Can you work these out from the model? Positions are in its coordinate system, mm. A direction names the side the tool comes from. Coordinates: 2 decimals unless noted, no trailing zeros. Order: outer loops, then holes, each group sorted by start corner. A loop starts at its lowest first (then second) coordinate and runs counter-clockwise, first axis right, second up.
```python
from build123d import *

# Parameters (mm, degrees)
SKETCH1_R                = 72.8
SKETCH1_R_2              = 2.065
SKETCH1_R_3              = 1.9558
SKETCH1_R_4              = 33.25
BOSS_EXTRUDE1_DEPTH      = 3.175
BOSS_EXTRUDE4_START      = 20
SKETCH14_R               = 72.8
SKETCH14_R_2             = 52.8
BOSS_EXTRUDE4_DEPTH      = 20
SKETCH15_R               = 2.065
CUT_EXTRUDE6_DEPTH       = 106.530851532
M5_CLEARANCE_HOLE1_D     = 5.3
CUT_EXTRUDE8_DEPTH       = 106.530851532
FILLET1_R                = 5
CIRPATTERN4_COUNT        = 3
FILLET1_OF_CIRPATTERN4_R = 5
BOSS_EXTRUDE8_START      = -20.175
BOSS_EXTRUDE8_DEPTH      = 30.175
CUT_EXTRUDE9_START       = -10
CUT_EXTRUDE9_DEPTH       = 10
CIRPATTERN5_COUNT        = 3


with BuildPart() as part:
    # Sketch1 → Boss-Extrude1 (new body)
    with BuildSketch(Plane.XY):
        Circle(SKETCH1_R)
        with Locations((50.662486121, -29.25)):
            Circle(SKETCH1_R_2, mode=Mode.SUBTRACT)
        with Locations((59.322740159, -34.25)):
            Circle(SKETCH1_R_2, mode=Mode.SUBTRACT)
        with Locations((-59.322740159, -34.25)):
            Circle(SKETCH1_R_2, mode=Mode.SUBTRACT)
        with Locations((-50.662486121, -29.25)):
            Circle(SKETCH1_R_2, mode=Mode.SUBTRACT)
        with Locations((0, 44.45)):
            Circle(SKETCH1_R_3, mode=Mode.SUBTRACT)
        with Locations((-44.45, 0)):
            Circle(SKETCH1_R_3, mode=Mode.SUBTRACT)
        with Locations((0, -44.45)):
            Circle(SKETCH1_R_3, mode=Mode.SUBTRACT)
        with Locations((31.430896424, -31.430896424)):
            Circle(SKETCH1_R_3, mode=Mode.SUBTRACT)
        with Locations((44.45, 0)):
            Circle(SKETCH1_R_3, mode=Mode.SUBTRACT)
        with Locations((0, 68.5)):
            Circle(SKETCH1_R_2, mode=Mode.SUBTRACT)
        with Locations((0, 58.5)):
            Circle(SKETCH1_R_2, mode=Mode.SUBTRACT)
        Circle(SKETCH1_R_4, mode=Mode.SUBTRACT)
    extrude(amount=BOSS_EXTRUDE1_DEPTH)

    # Sketch14 → Boss-Extrude4 (add)
    with BuildSketch(Plane(origin=(0, 0, 0), x_dir=(-1, 0, 0), z_dir=(0, 0, -1)).offset(BOSS_EXTRUDE4_START)):
        Circle(SKETCH14_R)
        Circle(SKETCH14_R_2, mode=Mode.SUBTRACT)
    extrude(amount=-BOSS_EXTRUDE4_DEPTH)

    # Sketch15 → Cut-Extrude6 (cut, through all)
    with BuildSketch(Plane.XY.offset(3.175)):
        with Locations((-59.322740159, -34.25)):
            Circle(SKETCH15_R)
        with Locations((-50.662486121, -29.25)):
            Circle(SKETCH15_R)
        with Locations((59.322740159, -34.25)):
            Circle(SKETCH15_R)
        with Locations((50.662486121, -29.25)):
            Circle(SKETCH15_R)
        with Locations((0, 58.5)):
            Circle(SKETCH15_R)
        with Locations((0, 68.5)):
            Circle(SKETCH15_R)
    extrude(amount=-CUT_EXTRUDE6_DEPTH, mode=Mode.SUBTRACT)

    # M5 Clearance Hole1 (through all)
    with Locations(Plane.XY.offset(3.175)):
        with Locations((0, 58.5), (0, 68.5), (50.662486121, -29.25), (59.322740159, -34.25), (-59.322740159, -34.25), (-50.662486121, -29.25)):
            Hole(M5_CLEARANCE_HOLE1_D / 2)

    # Sketch30 → Cut-Extrude8 (cut, through all)
    with BuildSketch(Plane(origin=(0, 0, -20), x_dir=(-1, 0, 0), z_dir=(0, 0, -1))):
        with BuildLine():
            ThreePointArc((-21.891382204, 69.430594014), (-63.046649396, 36.4), (-71.074349318, -15.756803895))
            Line((-71.074349318, -15.756803895), (-56.429909212, -12.510209686))
            Line((-56.429909212, -12.510209686), (-54.477317197, -12.077330458))
            ThreePointArc((-54.477317197, -12.077330458), (-48.324217531, 27.9), (-16.779383612, 53.217405852))
            Line((-16.779383612, 53.217405852), (-17.380795211, 55.124839753))
            Line((-17.380795211, 55.124839753), (-21.891382204, 69.430594014))
        make_face()
    cut_extrude8 = extrude(amount=-CUT_EXTRUDE8_DEPTH, mode=Mode.SUBTRACT)

    # Fillet1
    fillet1_edges = [part.edges().sort_by_distance(p)[0] for p in [
        (54.477317197, -12.077330458, -8.4125),
        (16.779383612, 53.217405852, -8.4125),
    ]]
    fillet(fillet1_edges, radius=FILLET1_R)

    # CirPattern4: Cut-Extrude8 ×3 about axis
    cirpattern4_axis = Axis((0, 0, 0), (0, 0, 1))
    for i in range(1, CIRPATTERN4_COUNT):
        add(cut_extrude8.rotate(cirpattern4_axis, i * 360 / CIRPATTERN4_COUNT), mode=Mode.SUBTRACT)

    # Fillet1 of CirPattern4
    fillet1_of_cirpattern4_edges = [part.edges().sort_by_distance(p)[0] for p in [
        (-16.779383612, 53.217405852, -8.4125),
        (-54.477317197, -12.077330458, -8.4125),
        (-37.697933585, -41.140075394, -8.4125),
        (37.697933585, -41.140075394, -8.4125),
    ]]
    fillet(fillet1_of_cirpattern4_edges, radius=FILLET1_OF_CIRPATTERN4_R)

    # Sketch31 → Boss-Extrude8 (add)
    with BuildSketch(Plane.XY.offset(3.175).offset(BOSS_EXTRUDE8_START)):
        with BuildLine():
            Line((21.891382204, 69.430594014), (21.816905179, 69.19438307))
            ThreePointArc((21.816905179, 69.19438307), (0, 72.552325945), (-21.816905179, 69.19438307))
            Line((-21.816905179, 69.19438307), (-22.883711342, 72.577859952))
            ThreePointArc((-22.883711342, 72.577859952), (0, 76.1), (22.883711342, 72.577859952))
            Line((22.883711342, 72.577859952), (21.891382204, 69.430594014))
        make_face()
    boss_extrude8 = extrude(amount=BOSS_EXTRUDE8_DEPTH)

    # Sketch32 → Cut-Extrude9 (cut)
    with BuildSketch(Plane.XY.offset(13.175).offset(CUT_EXTRUDE9_START)):
        with BuildLine():
            Line((21.816905179, 69.19438307), (22.883711342, 72.577859952))
            ThreePointArc((22.883711342, 72.577859952), (0, 76.1), (-22.883711342, 72.577859952))
            Line((-22.883711342, 72.577859952), (-21.816905179, 69.19438307))
            ThreePointArc((-21.816905179, 69.19438307), (0, 72.552325945), (21.816905179, 69.19438307))
        make_face()
    cut_extrude9 = extrude(amount=CUT_EXTRUDE9_DEPTH, mode=Mode.SUBTRACT)

    # CirPattern5: Boss-Extrude8, Cut-Extrude9 ×3 about axis
    cirpattern5_axis = Axis((0, 0, 0), (0, 0, 1))
    add([boss_extrude8.rotate(cirpattern5_axis, i * 360 / CIRPATTERN5_COUNT) for i in range(1, CIRPATTERN5_COUNT)])
    add([cut_extrude9.rotate(cirpattern5_axis, i * 360 / CIRPATTERN5_COUNT) for i in range(1, CIRPATTERN5_COUNT)], mode=Mode.SUBTRACT)


solid = part.part
```
1. Please list where these lines run through material, in increasing order: probe 1 along X at (y, z) = (-33, -1); probe 2 along X at (y, z) = (-49, -9.75); probe 3 along X at (y, z) = (24, -17) (3 decimals).
Completed:
probe 1: x = -68.57 to -61.66, -56.99 to -41.22, 41.22 to 56.99, 61.66 to 68.57
probe 2: x = -58.23 to -44.9, -26.7 to -19.67, 19.67 to 26.7, 44.9 to 58.23
probe 3: x = -50.375 to -47.03, 47.03 to 50.375
2. On a 3-axis mill with a long thin cutter (end or side, diameter ignored), from which of +Z, -Z, +X, -X, +Y, -Y can I reach the whole of each face in a straight line? I mean faces 4 (the flat face through (-24, 24, 0)), 5 (the cylindrical face through (-65.74, -38.33, -7.05)), 6 (the flat face through (-64, -36, -17)). Say none if no direction works.
Completed:
face 4: -Z
face 5: +Z, -Z, -X, -Y
face 6: -Z, -X, -Y
3. I'm going to push flat-ended pins straight in: pin 1 (6 mm diameter, centred on x = -18, z = 0, fed in from +Y); pin 2 (10 mm diameter, centred on y = -37, z = -10, fed in from -X) (3 decimals); pin 3 (8 mm diameter, centred on y = 3.5, z = -6, fed in from -X). Where does each tip first touch, or does it pass through?
Completed:
pin 1: stops at y = 74.61
pin 2: stops at x = -69.045
pin 3: stops at x = -55.8
4. Thinking about a two-plate mould opening in Y: for faces 1 (the flat face through (0, 74, -17)), 2 (the cylindrical face through (-53, -28, -9)), 3 (the cylindrical face through (-0.3, 72.8, -18.5)), which applies, pulls with the +Y half, pulls with the -Y half, needs draft (parallel to the pull), parting line crosses it, or undercut?
Completed:
face 1: needs draft
face 2: undercut
face 3: pulls with the +Y half
5. Imagine slicing it at B-B on x = 27.5. Please give me the cut outline in (y, z) (3 decimals).
Completed:
outline: (-48.553, -20) - (-45.073, -20) - (-45.073, 0) - (-18.69, 0) - (-18.69, 3.175) - (-48.553, 3.175) - close; (18.69, 0) - (45.073, 0) - (45.073, -20) - (48.553, -20) - (48.553, 3.175) - (18.69, 3.175) - close
6. Imagine slicing it at A-A on x = 0. Give the number of separate pieces and of enclosed holes in the cut face, then the cut area to 3 significant figures.
Completed:
separate pieces: 6
enclosed holes: 0
area: 453 mm2
7. Imagine slicing it at C-C on y = 26. Please give me the cut outline in (x, z) (3 decimals), then the cut area to 3 significant figures.
Completed:
outline: (-49.372, -20) - (-45.955, -20) - (-45.955, 0) - (-20.726, 0) - (-20.726, 3.175) - (-49.372, 3.175) - close; (20.726, 0) - (45.955, 0) - (45.955, -20) - (49.372, -20) - (49.372, 3.175) - (20.726, 3.175) - close
area: 319 mm2
